Source: CAD feature listing. Evaluate the final solid. Frame: model axes, mm. A direction names the side the tool comes from. Give positions to 0.01 mm unless a question says otherwise; leave off trailing zeros. Loops run counter-clockwise (first coordinate to the right, second up) from the corner with the lowest first, then second, coordinate; pieces in that order, holes last. Notation, with made-up numbers: (-8, 79) - (5, 79) arc R26 cw to (5, 104) - close; hole circle Ø10 at (37, 36). An arc over 180 degrees is marked (long way). Put each result on its own line as item: value.
```python
from build123d import *

# Parameters (mm, degrees)
SKETCH1_W           = 11.5
SKETCH1_H           = 66.675
SKETCH1_W_2         = 3.175
BOSS_EXTRUDE1_DEPTH = 3.175


with BuildPart() as part:
    # Sketch1 → Boss-Extrude1 (new body)
    with BuildSketch(Plane(origin=(0, 0, 0), x_dir=(1, 0, 0), z_dir=(0, 1, 0))):
        Polygon((-52.96, 85.881432482), (52.96, 85.881432482), (52.96, 82.706432482), (65.66, 82.706432482), (65.66, -47.723567518), (62.485, -47.723567518), (62.485, -60.423567518), (65.66, -60.423567518), (65.66, -72.868567518), (62.485, -72.868567518), (62.485, -85.568567518), (-62.485, -85.568567518), (-62.485, -72.868567518), (-65.66, -72.868567518), (-65.66, -60.423567518), (-62.485, -60.423567518), (-62.485, -47.723567518), (-65.66, -47.723567518), (-65.66, 82.706432482), (-52.96, 82.706432482), align=None)
        Polygon((-52.96, 6.506432482), (-14.097750884, 6.506432482), (-52.96, 62.098375408), align=None, mode=Mode.SUBTRACT)
        Polygon((-45.212249116, 73.181432482), (-6.35, 73.181432482), (-6.35, 17.589489555), align=None, mode=Mode.SUBTRACT)
        with Locations((-34.0045, -39.531067518)):
            Rectangle(SKETCH1_W, SKETCH1_H, mode=Mode.SUBTRACT)
        Polygon((52.96, 62.098375408), (52.96, 6.506432482), (14.097750884, 6.506432482), align=None, mode=Mode.SUBTRACT)
        Polygon((6.35, 73.181432482), (6.35, 17.589489555), (45.212249116, 73.181432482), align=None, mode=Mode.SUBTRACT)
        Polygon((14.097750884, -6.193567518), (52.96, -6.193567518), (52.96, -61.785510445), align=None, mode=Mode.SUBTRACT)
        Polygon((6.35, -17.276624592), (45.212249116, -72.868567518), (6.35, -72.868567518), align=None, mode=Mode.SUBTRACT)
        with Locations((-7.9375, -39.531067518)):
            Rectangle(SKETCH1_W_2, SKETCH1_H, mode=Mode.SUBTRACT)
    extrude(amount=BOSS_EXTRUDE1_DEPTH)


solid = part.part
```
1) Material intervals for line 1 along X through (y, z) = (1.5, -54); line 2 along Z through (x, y) = (-7.5, 3); line 3 along X through (y, z) = (0.7, -68), sorted ascending. Write a range as [from, to].
Check result:
line 1: [-65.66, -52.96], [-47.3, -31.8], [-6.35, 6.35], [31.8, 47.3], [52.96, 65.66]
line 2: [-85.88, -73.18], [-19.23, 6.19], [72.87, 85.57]
line 3: [-65.66, -41.59], [-6.35, 6.35], [41.59, 65.66]
2) Section query B-B, the plane x = -20. Output: boundary loops of the cut face in (y, z) (3 decimals).
Check result:
outline: (0, -85.881) - (3.175, -85.881) - (3.175, -73.181) - (0, -73.181) - close; (0, -37.116) - (3.175, -37.116) - (3.175, -14.95) - (0, -14.95) - close; (0, -6.506) - (3.175, -6.506) - (3.175, 85.569) - (0, 85.569) - close
3) Pin query (flat end, axial travel): P1, Ø1, axis at x = 64.5, y = 2, coming from the +Z side; P2, Ø1.6, axis at y = 1.5, z = 80.5, coming from the +X side (3 decimals). Return the tip coordinate at first contact, or that it passes through.
Check result:
P1: z = 72.87
P2: x = 62.485
4) Mould query, pull axis Z, two halves, no side actions, for faces 3 (the flat face through (25.51, 1.57, -45)), 4 (the flat face through (1, 0, -1)). Classes: pulls with the +Z half, pulls with the -Z half, needs draft (parallel to the pull), parting line crosses it, or undercut.
Check result:
face 3: undercut
face 4: needs draft
5) Access query for faces 1 (the flat face through (33.257, 1.565, -33.913)), 2 (the flat face through (1, 3.175, -1)). Directions: +Z, -Z, +X, -X, +Y, -Y. A direction counts if a zero-diameter tool reaches every point of the face in a straight line with its end or side. Return the directions, or none.
Check result:
face 1: +Y, -Y
face 2: +Z, -Z, +X, -X, +Y
6) Section query A-A, the plane z = 36. State how many separate pieces and enclosed holes the cut face has, plus the area to 3 significant figures.
Check result:
separate pieces: 5
enclosed holes: 0
area: 272 mm²
